```python
from build123d import *

# Parameters (mm, degrees)
PAD_DEPTH       = 9
SKETCH001_R     = 2
POCKET_DEPTH    = 135.76007
SKETCH002_R     = 2
POCKET001_DEPTH = 98.114621
SKETCH003_R     = 5
POCKET002_DEPTH = 93.114621
SKETCH004_R     = 5
POCKET003_DEPTH = 130.76007
CHAMFER_SIZE    = 1


with BuildPart() as part:
    # Sketch → Pad (new body, symmetric)
    with BuildSketch(Plane.XY):
        with BuildLine():
            Line((65.879535, 49.056811), (-65.879535, 49.056811))
            ThreePointArc((-65.879535, 49.056811), (-67.293749, 48.471024), (-67.879535, 47.056811))
            Line((-67.879535, 47.056811), (-67.879535, -47.056811))
            ThreePointArc((-67.879535, -47.056811), (-66.794698, -48.835146), (-64.717059, -48.684278))
            Line((-64.717059, -48.684278), (67.042011, 45.429344))
            ThreePointArc((67.042011, 45.429344), (67.784126, 47.667166), (65.879535, 49.056811))
        make_face()
    extrude(amount=PAD_DEPTH, both=True)

    # Sketch001 (on Face3 of Pad) → Pocket (cut, through all)
    with BuildSketch(Plane(origin=(-67.879535, 0, 0), x_dir=(0, -1, 0), z_dir=(-1, 0, 0))):
        with Locations((26.943189, 0)):
            Circle(SKETCH001_R)
    extrude(amount=-POCKET_DEPTH, mode=Mode.SUBTRACT)

    # Sketch002 (on Face1 of Pocket) → Pocket001 (cut, through all)
    with BuildSketch(Plane(origin=(0, 49.056811, 0), x_dir=(-1, 0, 0), z_dir=(0, 1, 0))):
        with Locations((-47.120465, 0)):
            Circle(SKETCH002_R)
    extrude(amount=-POCKET001_DEPTH, mode=Mode.SUBTRACT)

    # Sketch003 (on Face1 of Pocket001) → Pocket002 (cut, through all)
    with BuildSketch(Plane(origin=(0, 44.056811, 0), x_dir=(-1, 0, 0), z_dir=(0, 1, 0))):
        with Locations((-47.120465, 0)):
            Circle(SKETCH003_R)
    extrude(amount=-POCKET002_DEPTH, mode=Mode.SUBTRACT)

    # Sketch004 (on Face8 of Pocket002) → Pocket003 (cut, through all)
    with BuildSketch(Plane(origin=(-62.879535, 0, 0), x_dir=(0, -1, 0), z_dir=(-1, 0, 0))):
        with Locations((26.943189, 0)):
            Circle(SKETCH004_R)
    extrude(amount=-POCKET003_DEPTH, mode=Mode.SUBTRACT)

    # Chamfer
    chamfer_edges = [part.edges().sort_by_distance(p)[0] for p in [
        (0, 49.056811, 9),
        (-67.293749, 48.471024, 9),
        (-67.879535, 0, 9),
        (-66.794698, -48.835146, 9),
        (1.162476, -1.627467, 9),
        (67.784126, 47.667166, 9),
        (0, 49.056811, -9),
        (-67.293749, 48.471024, -9),
        (-67.879535, 0, -9),
        (-66.794698, -48.835146, -9),
        (1.162476, -1.627467, -9),
        (67.784126, 47.667166, -9),
    ]]
    chamfer(chamfer_edges, length=CHAMFER_SIZE)


solid = part.part
```
The model under review builds one solid part; all positions refer to its coordinate system, in mm. A direction names the side the tool comes from. Give positions to 0.01 mm unless a question says otherwise; leave off trailing zeros. Write each loop counter-clockwise with the first axis right and the second up, starting at its lowest first coordinate (ties: lowest second). Pieces come first, ordered by that corner, then holes. Notation, with made-up numbers: (6, -20.5) -> (31, -20.5) arc R20 cw to (31, 11.5) -> close; hole circle Ø2 at (-9, 62). An arc over 180 degrees is marked (long way). Answer in a Markdown table with one row per item.
1) Add section B-B on x = -54. State the section outline as (y, z) points.
Worked answers:
| item | result |
|---|---|
| outline | (-41.03, -8) -> (-39.8, -9) -> (48.06, -9) -> (49.06, -8) -> (49.06, 8) -> (48.06, 9) -> (-39.8, 9) -> (-41.03, 8) -> close; hole circle Ø10 at (-26.94, 0) |
2) Add section D-D on x = -10. State the section outline as (y, z) points, plus the area to 3 significant figures.
Worked answers:
| item | result |
|---|---|
| outline | (-9.6, -8) -> (-8.37, -9) -> (48.06, -9) -> (49.06, -8) -> (49.06, 8) -> (48.06, 9) -> (-8.37, 9) -> (-9.6, 8) -> close |
| area | 1,050 mm² |
3) Mouldability with a two-part tool opening along X and no side actions: class faces 4 (the flat face through (-62.88, -29.1, 0.1)), 5 (the flat face through (44.97, 44.057, 0.07)), 6 (the cylindrical face through (-65.415, -24.945, 0.088)), 7 (the cylindrical face through (45.273, 46.592, -0.766)) as +X half, -X half, draft (parallel to the pull), parting line (faces both ways), or undercut.
Worked answers:
| item | result |
|---|---|
| face 4 | +X half |
| face 5 | undercut |
| face 6 | draft |
| face 7 | undercut |
4) Add section C-C on y = 13. State the section outline as (x, z) points.
Worked answers:
| item | result |
|---|---|
| outline | (-67.88, -8) -> (-66.88, -9) -> (19.92, -9) -> (21.64, -8) -> (21.64, 8) -> (19.92, 9) -> (-66.88, 9) -> (-67.88, 8) -> close |
5) For L1, parallel to Y at x = -52.5, z = 0; L2, parallel to Y at x = -61, z = 2.5; L3, parallel to Y at x = 44, z = -3.25, list the stretches that pass through material, from the lowest coordinate up. Write a range as [from, to].
Worked answers:
| item | result |
|---|---|
| L1 | [-39.96, -31.94], [-21.94, 49.06] |
| L2 | [-46.03, -31.27], [-22.61, 49.06] |
| L3 | [44.06, 49.06] |
6) Add section A-A on z = 0. State the section outline as (x, y) points, plus the area to 3 significant figures.
Worked answers:
| item | result |
|---|---|
| outline | (-67.88, -47.06) arc R2 ccw to (-64.72, -48.68) -> (-41.28, -31.94) -> (-62.88, -31.94) -> (-62.88, -28.94) -> (-67.88, -28.94) -> close; (-67.88, -24.94) -> (-62.88, -24.94) -> (-62.88, -21.94) -> (-27.28, -21.94) -> (42.12, 27.63) -> (42.12, 44.06) -> (45.12, 44.06) -> (45.12, 49.06) -> (-65.88, 49.06) arc R2 ccw to (-67.88, 47.06) -> close; (49.12, 44.06) -> (52.12, 44.06) -> (52.12, 34.77) -> (67.04, 45.43) arc R2 ccw to (65.88, 49.06) -> (49.12, 49.06) -> close |
| area | 6,530 mm² |
7) Clearance check with flat-ended pins moving along their axes: P1, Ø5, axis at x = 49, z = 5, coming from the -Y side; P2, Ø8, axis at y = -26.94, z = 0, coming from the +X side; P3, Ø8, axis at y = -24.5, z = -2, coming from the +X side; P4, Ø3, axis at x = 47.12, z = 0, coming from the -Y side. State where each tip first meets the part, or that it passes through.
Worked answers:
| item | result |
|---|---|
| P1 | y = 30.76 |
| P2 | x = -62.88 |
| P3 | x = -25.26 |
| P4 | through |
8) Tool access review of faces 1 (the cylindrical face through (-49.17, -21.95, 0.22)), 2 (the cylindrical face through (42.35, 37.78, 1.5)), 3 (the flat face through (-16, 11, 9)): name each direction out of +Z, -Z, +X, -X, +Y, -Y from which nothing blocks a thin tool from reaching the whole face with its end or side.
Worked answers:
| item | result |
|---|---|
| face 1 | +X |
| face 2 | -Y |
| face 3 | +Z, +X, -X, +Y, -Y |
